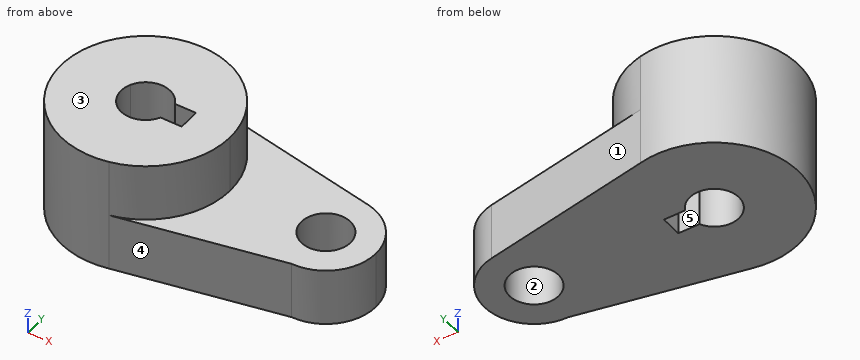
```python
from build123d import *

# Parameters (mm, degrees)
F0_R     = 10.795
F1_DEPTH = 25.4
F2_DEPTH = 50.8


with BuildPart() as f1:
    # F0 (on Top) → F1 (new body)
    with BuildSketch(Plane.XY):
        with BuildLine():
            ThreePointArc((-9.718612, -4.699), (-10.795, 0), (-9.718612, 4.699))
            Line((-9.718612, 4.699), (-19.05, 4.699))
            Line((-19.05, 4.699), (-19.05, -4.699))
            Line((-19.05, -4.699), (-9.718612, -4.699))
        make_face()
        with BuildLine():
            ThreePointArc((8.266151, -36.196979), (29.029839, -23.147764), (37.128837, 0))
            ThreePointArc((37.128837, 0), (29.029839, 23.147764), (8.266151, 36.196979))
            ThreePointArc((8.266151, 36.196979), (-37.128837, 0), (8.266151, -36.196979))
        make_face()
        with BuildLine():
            ThreePointArc((-9.718612, 4.699), (0, 10.795), (9.718612, 4.699))
            Line((9.718612, 4.699), (19.05, 4.699))
            Line((19.05, 4.699), (19.05, -4.699))
            Line((19.05, -4.699), (9.718612, -4.699))
            ThreePointArc((9.718612, -4.699), (0, -10.795), (-9.718612, -4.699))
            Line((-9.718612, -4.699), (-19.05, -4.699))
            Line((-19.05, -4.699), (-19.05, 4.699))
            Line((-19.05, 4.699), (-9.718612, 4.699))
        make_face(mode=Mode.SUBTRACT)
        with BuildLine():
            ThreePointArc((101.319549, 0), (96.309698, 13.956332), (83.567604, 21.540318))
            ThreePointArc((83.567604, 21.540318), (57.549179, 2.279634), (79.026044, -21.941774))
            ThreePointArc((79.026044, -21.941774), (94.76827, -15.640027), (101.319549, 0))
        make_face()
        with Locations((79.375, 0)):
            Circle(F0_R, mode=Mode.SUBTRACT)
        with BuildLine():
            ThreePointArc((8.266151, 36.196979), (29.029839, 23.147764), (37.128837, 0))
            ThreePointArc((37.128837, 0), (29.029839, -23.147764), (8.266151, -36.196979))
            Line((8.266151, -36.196979), (79.026044, -21.941774))
            ThreePointArc((79.026044, -21.941774), (57.549179, 2.279634), (83.567604, 21.540318))
            Line((83.567604, 21.540318), (8.266151, 36.196979))
        make_face()
    extrude(amount=F1_DEPTH)

    # F0 (on Top) → F2 (join)
    with BuildSketch(Plane.XY):
        with BuildLine():
            ThreePointArc((8.266151, -36.196979), (29.029839, -23.147764), (37.128837, 0))
            ThreePointArc((37.128837, 0), (29.029839, 23.147764), (8.266151, 36.196979))
            ThreePointArc((8.266151, 36.196979), (-37.128837, 0), (8.266151, -36.196979))
        make_face()
        with BuildLine():
            ThreePointArc((-9.718612, 4.699), (0, 10.795), (9.718612, 4.699))
            Line((9.718612, 4.699), (19.05, 4.699))
            Line((19.05, 4.699), (19.05, -4.699))
            Line((19.05, -4.699), (9.718612, -4.699))
            ThreePointArc((9.718612, -4.699), (0, -10.795), (-9.718612, -4.699))
            Line((-9.718612, -4.699), (-19.05, -4.699))
            Line((-19.05, -4.699), (-19.05, 4.699))
            Line((-19.05, 4.699), (-9.718612, 4.699))
        make_face(mode=Mode.SUBTRACT)
        with BuildLine():
            ThreePointArc((-9.718612, -4.699), (-10.795, 0), (-9.718612, 4.699))
            Line((-9.718612, 4.699), (-19.05, 4.699))
            Line((-19.05, 4.699), (-19.05, -4.699))
            Line((-19.05, -4.699), (-9.718612, -4.699))
        make_face()
    extrude(amount=F2_DEPTH)


solid = f1.part
```
Model file for the job. Use its own axes, mm. Face numbers are marked on the shaded views. A direction names the side the tool comes from. Coordinates: 2 decimals unless noted, no trailing zeros. Loops run counter-clockwise (first coordinate to the right, second up) from the corner with the lowest first, then second, coordinate; pieces in that order, holes last. Notation, with made-up numbers: (16.5, 25.25) - (75.5, 25.25) arc R35 ccw to (75.5, 59.25) - close; hole circle Ø3 at (17.5, 57.5). An arc over 180 degrees is marked (long way). Answer as a JSON object with one key per item and string values. Group by question number.
(1) Two-plate mould, pull along X, no slides. Class the marked faces 1, 2 and 3: released by +X, released by -X, zero draft, split by the parting line, or undercut.
(2) Tool access for the marked faces 4 and 5: list every direction of +Z, -Z, +X, -X, +Y, -Y with a clear straight run to the whole face (end or side of a thin tool).
(3) Cut at B-B (z = 36.5). Give the cut face in (x, y) (3 decimals).
(4) Cut at A-A (x = 0). Give the cut face in (y, z) (3 decimals), then the cut area to 3 significant figures.
(5) Flat gauge pins, fed straight in: pin 1 (12 mm diameter, centred on x = 4.5, y = 29, fed in from -Z); pin 2 (4 mm diameter, centred on y = 21, z = 26, fed in from -X); pin 3 (10.5 mm diameter, centred on x = 14.5, z = 18.5, fed in from +Y); pin 4 (6 mm diameter, centred on x = 50, z = 16, fed in from -Y). Where does each tip first touch, or does it go through?
(6) Probe line 1 along X through (y, z) = (0, 34.5) (3 decimals); line 2 along Z through (x, y) = (55, 6); line 3 along Y through (x, z) = (4.5, 17). List the from-to ranges inside material, lowest first.
(7) Cut at C-C (z = 18). Give the cut face in (x, y) (3 decimals).
(8) Cut at D-D (x = 32). Give the cut face in (y, z), then the cut area to 3 significant figures.
Geometry says:
{
 "1": {"face 1": "released by +X", "face 2": "undercut", "face 3": "zero draft"},
 "2": {"face 4": "+Z, -Z, +X, -Y", "face 5": "+Z, -Z"},
 "3": {"outline": "circle Ø74.258 at (0, 0); hole (-9.719, -4.699) arc R10.795 ccw to (9.719, -4.699) - (19.05, -4.699) - (19.05, 4.699) - (9.719, 4.699) arc R10.795 ccw to (-9.719, 4.699) arc R10.795 ccw to start"},
 "4": {"outline": "(-37.129, 0) - (-10.795, 0) - (-10.795, 50.8) - (-37.129, 50.8) - close; (10.795, 0) - (37.129, 0) - (37.129, 50.8) - (10.795, 50.8) - close", "area": "2,680 mm^2"},
 "5": {"pin 1": "stops at z = 0", "pin 2": "stops at x = -31.9", "pin 3": "stops at y = 36.01", "pin 4": "stops at y = -28.39"},
 "6": {"line 1": "x = -37.129 to -10.795, 19.05 to 37.129", "line 2": "z = 0 to 25.4", "line 3": "y = -36.86 to -9.81, 9.81 to 36.86"},
 "7": {"outline": "(8.266, -36.197) - (79.026, -21.942) arc R21.945 ccw to (101.32, 0) arc R21.945 ccw to (83.568, 21.54) - (8.266, 36.197) arc R37.129 ccw (long way) to start; hole (-9.719, -4.699) arc R10.795 ccw to (9.719, -4.699) - (19.05, -4.699) - (19.05, 4.699) - (9.719, 4.699) arc R10.795 ccw to (-9.719, 4.699) arc R10.795 ccw to start; hole circle Ø21.59 at (79.375, 0)"},
 "8": {"outline": "(-31.42, 0) - (31.58, 0) - (31.58, 25.4) - (18.83, 25.4) - (18.83, 50.8) - (-18.83, 50.8) - (-18.83, 25.4) - (-31.42, 25.4) - close", "area": "2,560 mm^2"}
}
